```python
from build123d import *

# Parameters (mm, degrees)
SKETCH1_R           = 7.5
BOSS_EXTRUDE1_DEPTH = 10
SKETCH5_R           = 6
BOSS_EXTRUDE2_DEPTH = 2
FILLET2_R           = 1
BOSS_EXTRUDE3_DEPTH = 6
CUT_EXTRUDE4_DEPTH  = 29
CUT_EXTRUDE5_START  = -1
SKETCH10_R          = 2
CUT_EXTRUDE5_DEPTH  = 20
CUT_EXTRUDE6_START  = -24
CUT_EXTRUDE6_DEPTH  = 24


with BuildPart() as part:
    # Sketch1 → Boss-Extrude1 (new body)
    with BuildSketch(Plane(origin=(0, 0, 0), x_dir=(1, 0, 0), z_dir=(0, 1, 0))):
        with Locations(Location((0, 0, 0), (0, 0, 270))):
            Circle(SKETCH1_R)
    boss_extrude1 = extrude(amount=BOSS_EXTRUDE1_DEPTH)

    # Sketch5 → Boss-Extrude2 (add)
    with BuildSketch(Plane(origin=(0, 10, 0), x_dir=(1, 0, 0), z_dir=(0, 1, 0))):
        with Locations(Location((0, 0, 0), (0, 0, 270))):
            Circle(SKETCH5_R)
    boss_extrude2 = extrude(amount=BOSS_EXTRUDE2_DEPTH)

    # Fillet2
    fillet2_edges = [part.edges().sort_by_distance(p)[0] for p in [
        (0, 10, -6),
    ]]
    fillet(fillet2_edges, radius=FILLET2_R)

    # Sketch6 → Boss-Extrude3 (add, symmetric)
    with BuildSketch(Plane(origin=(0, 0, 0), x_dir=(0, 0, -1), z_dir=(1, 0, 0))):
        Polygon((6, 12), (-6, 12), (-11, 12), (-11, 27), (-9, 27), (-9, 14), (9, 14), (9, 27), (11, 27), (11, 12), align=None)
    boss_extrude3 = extrude(amount=BOSS_EXTRUDE3_DEPTH, both=True)

    # Sketch9 → Cut-Extrude4 (cut)
    with BuildSketch(Plane.XY.offset(11)):
        with BuildLine():
            Line((-6, 27), (-6, 21))
            ThreePointArc((-6, 21), (-4.052343178, 25.052343178), (0, 27))
            Line((0, 27), (-6, 27))
        make_face()
        with BuildLine():
            ThreePointArc((0, 27), (4.052343178, 25.052343178), (6, 21))
            Line((6, 21), (6, 27))
            Line((6, 27), (0, 27))
        make_face()
    cut_extrude4 = extrude(amount=-CUT_EXTRUDE4_DEPTH, mode=Mode.SUBTRACT)

    # Sketch10 → Cut-Extrude5 (cut)
    with BuildSketch(Plane(origin=(0, 0, 9), x_dir=(-1, 0, 0), z_dir=(0, 0, -1)).offset(CUT_EXTRUDE5_START)):
        with Locations(Location((0, 24.25, 0), (0, 0, 180))):
            Circle(SKETCH10_R)
    cut_extrude5 = extrude(amount=CUT_EXTRUDE5_DEPTH, mode=Mode.SUBTRACT)

    # Mirror2: Boss-Extrude1 across plane
    add(boss_extrude1.mirror(Plane.ZX))

    # Mirror9: Boss-Extrude2, Boss-Extrude3 across plane
    add(boss_extrude2.mirror(Plane.ZX))
    add(boss_extrude3.mirror(Plane.ZX))

    # Mirror11: Cut-Extrude4, Cut-Extrude5 across plane
    add(cut_extrude4.mirror(Plane.ZX), mode=Mode.SUBTRACT)
    add(cut_extrude5.mirror(Plane.ZX), mode=Mode.SUBTRACT)

    # Sketch11 → Cut-Extrude6 (cut)
    with BuildSketch(Plane(origin=(0, 0, -11), x_dir=(-1, 0, 0), z_dir=(0, 0, -1)).offset(CUT_EXTRUDE6_START)):
        with BuildLine():
            Line((-4.052343178, 12), (-4.052343178, 25.052343178))
            ThreePointArc((-4.052343178, 25.052343178), (-5.371235948, 23.192018094), (-6, 21))
            Line((-6, 21), (-6, 12))
            Line((-6, 12), (-4.052343178, 12))
        make_face()
        with BuildLine():
            Line((4.052343178, 25.052343178), (4.052343178, 12))
            Line((4.052343178, 12), (6, 12))
            Line((6, 12), (6, 21))
            ThreePointArc((6, 21), (5.371235948, 23.192018094), (4.052343178, 25.052343178))
        make_face()
    cut_extrude6 = extrude(amount=CUT_EXTRUDE6_DEPTH, mode=Mode.SUBTRACT)

    # Mirror12: Cut-Extrude6 across plane
    add(cut_extrude6.mirror(Plane.ZX), mode=Mode.SUBTRACT)


solid = part.part
```
Input: part model. Units: mm. Frame: model coordinates. A direction names the side the tool comes from. Give positions to 0.01 mm unless a question says otherwise; leave off trailing zeros. Order: outer loops, then holes, each group sorted by start corner. A loop starts at its lowest first (then second) coordinate and runs counter-clockwise, first axis right, second up. Notation, with made-up numbers: M -11,89.5 L -1,89.5 A31 ccw -1,125.5 Z; hole C -7,5.25 d8. An arc over 180 degrees is marked long. Return JSON: item names as keys, results as strings.
1) Line query: L1, parallel to Z at x = -2.75, y = -17; L2, parallel to Y at x = -1, z = 6.25; L3, parallel to X at y = 24.25, z = -9.7. Output: solid intervals per line, ascending. Write a range as [from, to].
Taken from the geometry:
{"L1": "z = [-11, -9], [9, 11]", "L2": "y = [-14, -12], [-10, 10.26], [12, 14]", "L3": "x = [-4.05, -2], [2, 4.05]"}
2) Mould query, pull axis Y, two halves, no side actions, for faces 6 (the face through (0, 19, 9)), 7 (the face through (0.33, 0.14, -7.493)), 8 (the face through (5, -12, 0)). Classes: released by +Y, released by -Y, zero draft, split by the parting line, or undercut.
Taken from the geometry:
{"face 6": "zero draft", "face 7": "undercut", "face 8": "released by -Y"}
3) Section query A-A on z = 8.25. Output: boundary loops of the cut face in (x, y).
Taken from the geometry:
{"outline": "M -4.05,-14 L 4.05,-14 L 4.05,-12 L -4.05,-12 Z; M -4.05,12 L 4.05,12 L 4.05,14 L -4.05,14 Z"}
4) Section query C-C on z = 0. Output: boundary loops of the cut face in (x, y).
Taken from the geometry:
{"outline": "M -7.5,-10 L -6,-10 L -6,-12 L -4.05,-12 L -4.05,-14 L 4.05,-14 L 4.05,-12 L 6,-12 L 6,-10 L 7.5,-10 L 7.5,10 L 7,10 A1 cw 6,11 L 6,12 L 4.05,12 L 4.05,14 L -4.05,14 L -4.05,12 L -6,12 L -6,11 A1 cw -7,10 L -7.5,10 Z"}
5) Section query B-B on y = -24.25. Output: boundary loops of the cut face in (x, z).
Taken from the geometry:
{"outline": "M -4.05,-11 L 4.05,-11 L 4.05,-9 L 2,-9 L 2,-10 L -2,-10 L -2,-9 L -4.05,-9 Z; M -4.05,9 L -2,9 L -2,10 L 2,10 L 2,9 L 4.05,9 L 4.05,11 L -4.05,11 Z"}
6) Section query D-D on y = -9.5. Output: boundary loops of the cut face in (x, z).
Taken from the geometry:
{"outline": "C 0,0 d15"}
7) Access query for faces 1 (the face through (-2.221, 26.357, -9.986)), 2 (the face through (0, -19, -9)), 3 (the face through (5, 12, 0)), 4 (the face through (0, -24, 10)), 5 (the face through (0, 14, 0)). Directions: +Z, -Z, +X, -X, +Y, -Y. A direction counts if a zero-diameter tool reaches every point of the face in a straight line with its end or side. Return the directions, or none.
Taken from the geometry:
{"face 1": "+Z, -Z, -X, +Y", "face 2": "+X, -X, -Y", "face 3": "+Z, -Z, +X, +Y", "face 4": "none", "face 5": "+X, -X, +Y"}
8) Contact query for flat-ended pins moving along their axis: pin 1 (2 mm diameter, centred on x = 5.5, z = 2, fed in from -Y); pin 2 (12 mm diameter, centred on y = -9.5, z = 4.5, fed in from -X); pin 3 (10.5 mm diameter, centred on y = -17.5, z = 5, fed in from +X); pin 4 (1 mm diameter, centred on x = 5.5, z = -2, fed in from +Y). Output: stop coordinate, or through.
Taken from the geometry:
{"pin 1": "stops at y = -12", "pin 2": "stops at x = -7.5", "pin 3": "stops at x = 4.05", "pin 4": "stops at y = 12"}
